Source: CAD feature listing. Evaluate the final solid. Frame: model axes, mm. Face numbers are marked on the shaded views. A direction names the side the tool comes from. Round coordinates to 2 decimals unless told otherwise and drop trailing zeros. Loops run counter-clockwise (first coordinate to the right, second up) from the corner with the lowest first, then second, coordinate; pieces in that order, holes last. Notation, with made-up numbers: (86, 47.5) - (102, 47.5) arc R21 cw to (102, 67.5) - close; hole circle Ø11 at (31.5, 39.25). An arc over 180 degrees is marked (long way). Use CSV: the item, a comma, the result in double quotes. Start each with the question number.
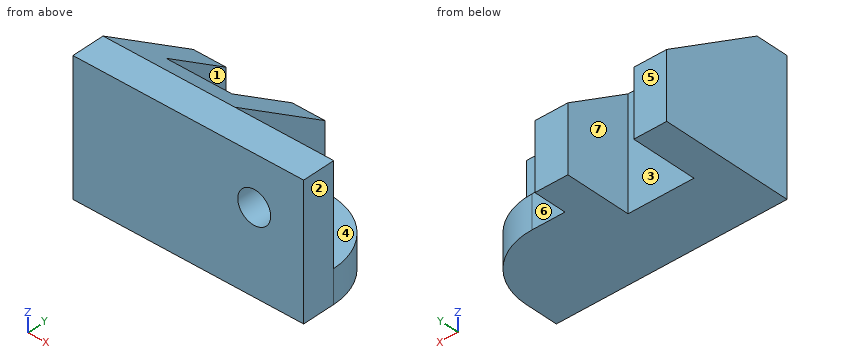
from build123d import *

# Parameters (mm, degrees)
SKETCH_1_W          = 15
SKETCH_1_H          = 15
SKETCH_1_R          = 2.5
EXTRUDE_1_DEPTH     = 5
SKETCH_1_3_W        = 15
SKETCH_1_3_H        = 5
EXTRUDE_2_DEPTH     = 15
EXTRUDE_3_DEPTH     = 20
CUT_EXTRUDE_1_DEPTH = 20
SKETCH_3_W          = 10
SKETCH_3_H          = 10
CUT_EXTRUDE_2_DEPTH = 20
FILLET_1_R          = 10


with BuildPart() as part:
    # 草圖1 → 填料-伸長1 (new body)
    with BuildSketch(Plane(origin=(0, 0, 0), x_dir=(1, 0, 0), z_dir=(0, 1, 0))):
        with Locations((10, -2.5)):
            Rectangle(SKETCH_1_W, SKETCH_1_H)
        with Locations((10, -2.5)):
            Circle(SKETCH_1_R, mode=Mode.SUBTRACT)
    extrude(amount=EXTRUDE_1_DEPTH)

    # 草圖1<3> → 填料-伸長2 (add)
    with BuildSketch(Plane(origin=(0, 0, 0), x_dir=(1, 0, 0), z_dir=(0, 1, 0))):
        with Locations((10, 7.5)):
            Rectangle(SKETCH_1_3_W, SKETCH_1_3_H)
    extrude(amount=EXTRUDE_2_DEPTH)

    # 草圖1<4> → 填料-伸長3 (add)
    with BuildSketch(Plane(origin=(0, 0, 0), x_dir=(1, 0, 0), z_dir=(0, 1, 0))):
        Polygon((-17.5, 10), (-17.5, -10), (2.5, -10), (2.5, 5), (2.5, 10), align=None)
    extrude(amount=EXTRUDE_3_DEPTH)

    # 草圖2 → 除料-伸長1 (cut)
    with BuildSketch(Plane(origin=(2.5, 0, 0), x_dir=(0, 0, -1), z_dir=(1, 0, 0))):
        Polygon((-10, 5), (0, 20), (-10, 20), align=None)
    extrude(amount=-CUT_EXTRUDE_1_DEPTH, mode=Mode.SUBTRACT)

    # 草圖3 → 除料-伸長2 (cut)
    with BuildSketch(Plane(origin=(0, 0, -10), x_dir=(-1, 0, 0), z_dir=(0, 0, -1))):
        with Locations((7.5, 15)):
            Rectangle(SKETCH_3_W, SKETCH_3_H)
    extrude(amount=-CUT_EXTRUDE_2_DEPTH, mode=Mode.SUBTRACT)

    # 圓角1
    fillet_1_edges = [part.edges().sort_by_distance(p)[0] for p in [
        (17.5, 15, -7.5),
    ]]
    fillet(fillet_1_edges, radius=FILLET_1_R)


solid = part.part
1. Reachability of the marked faces 5, 6 and 7 from +Z, -Z, +X, -X, +Y, -Y: full face, straight path, thin tool, end or side. Return the list, or none.
2. Contact query for flat-ended pins moving along their axis: P1, Ø6, axis at x = 0, z = 2, coming from the -Y side; P2, Ø6, axis at x = 10, z = 2.5, coming from the +Y side; P3, Ø7.5, axis at y = 15.5, z = -4.5, coming from the +X side; P4, Ø11, axis at y = 15.5, z = -5.5, coming from the +X side. Output: stop coordinate, or through.
3. Section query B-B on z = -1.5. Return the cut outline in (x, y), and give its area (3 significant figures).
4. Section query C-C on z = 2.5. Return the cut outline in (x, y), and give its area (4 significant figures).
5. Section query D-D on x = -14. Return the cut outline in (y, z), and give its area (3 significant figures).
6. Section query A-A on y = 11. Return the cut outline in (x, z).
7. Line query: line 1 along X through (y, z) = (1.55, 2.5); line 2 along Z through (x, y) = (10, 1.9); line 3 along X through (y, z) = (13.5, -2). Output: solid intervals per line, ascending.
8. Mould query, pull axis X, two halves, no side actions, for the marked faces 1, 2, 3 and 4. Classes: +X half, -X half, draft (parallel to the pull), parting line (faces both ways), or undercut.
Values:
1,face 5,"+Z, -Z, +X, -X, +Y"
1,face 6,"+Z, -Z, +X, +Y"
1,face 7,"+Z, -Z, +Y"
2,P1,"stops at y = 0"
2,P2,"stops at y = 5"
2,P3,"stops at x = 14.85"
2,P4,"stops at x = 16.16"
3,outline,"(-17.5, 0) - (17.5, 0) - (17.5, 5) - (2.5, 5) - (2.5, 20) - (-2.5, 20) - (-2.5, 10) - (-12.5, 10) - (-12.5, 20) - (-17.5, 20) - close"
3,area,"375 mm^2"
4,outline,"(-17.5, 0) - (7.5, 0) - (7.5, 5) - (2.5, 5) - (2.5, 16.25) - (-2.5, 16.25) - (-2.5, 10) - (-12.5, 10) - (-12.5, 16.25) - (-17.5, 16.25) - close; (12.5, 0) - (17.5, 0) - (17.5, 5) - (12.5, 5) - close"
4,area,"312.5 mm^2"
5,outline,"(0, -10) - (20, -10) - (20, 0) - (5, 10) - (0, 10) - close"
5,area,"325 mm^2"
6,outline,"(-17.5, -10) - (-12.5, -10) - (-12.5, 6) - (-17.5, 6) - close; (-2.5, -10) - (15.5, -10) - (15.5, -5) - (2.5, -5) - (2.5, 6) - (-2.5, 6) - close"
7,line 1,"x = -17.5 to 7.5, 12.5 to 17.5"
7,line 2,"z = -10 to 0, 5 to 10"
7,line 3,"x = -17.5 to -12.5, -2.5 to 2.5"
8,face 1,"undercut"
8,face 2,"+X half"
8,face 3,"undercut"
8,face 4,"draft"
